Source: CAD feature listing. Evaluate the final solid. Frame: model axes, mm. A direction names the side the tool comes from. Coordinates: 2 decimals unless noted, no trailing zeros. Order: outer loops, then holes, each group sorted by start corner. A loop starts at its lowest first (then second) coordinate and runs counter-clockwise, first axis right, second up. Notation, with made-up numbers: (-27, 46) -> (7, 46) arc R13 cw to (7, 65) -> close; hole circle Ø11 at (-37.75, -30). An arc over 180 degrees is marked (long way). Write item = value, one per line. Start each with the question number.
Item 1: Contact query for flat-ended pins moving along their axis: pin 1 (6 mm diameter, centred on x = -4, z = -4, fed in from -Y); pin 2 (3 mm diameter, centred on x = 4, z = 4, fed in from -Y). Output: stop coordinate, or through.
Item 2: Section query C-C (x = -4). Output: boundary loops of the cut face in (y, z).
Item 3: Ray query, line 1 along X through (y, z) = (1.05, -4); line 2 along X through (y, z) = (1.05, 3.5); line 3 along Z through (x, y) = (-6, 1.4). Return the intervals inside material, ascending. Write a range as [from, to].
Item 4: Section query B-B (z = -4). Output: boundary loops of the cut face in (x, y).
Item 5: Set-up query: faces 4 (the cylindrical face through (-3.249, 0.887, 6.385)), 5 (the flat face through (0, 0, 0)). Return all of +Z, -Z, +X, -X, +Y, -Y with unobstructed straight access to the full face (end or side cutting, diameter ignored); none if empty.
Item 6: Section query A-A (y = 0.95). Output: boundary loops of the cut face in (x, z), then the cut area to 3 significant figures.
Item 7: Mould query, pull axis Z, two halves, no side actions, for faces 1 (the flat face through (0, 2, -7.9)), 2 (the flat face through (-7.9, 2, 0)), 3 (the cylindrical face through (-3.249, 0.887, -1.615)). Classes: released by +Z, released by -Z, zero draft, split by the parting line, or undercut.
```python
from build123d import *

# Parameters (mm, degrees)
SKETCH_1_W          = 15.8
SKETCH_1_H          = 15.8
SKETCH_1_R          = 2.5
EXTRUDE_1_DEPTH     = 3.2
SKETCH_1_5_R        = 2.5
CUT_EXTRUDE_1_DEPTH = 1.8


with BuildPart() as part:
    # Sketch 1 → Extrude 1 (new body)
    # profile 1 of 5: a face of its own
    with BuildSketch(Plane(origin=(0, 0, 0), x_dir=(1, 0, 0), z_dir=(0, 1, 0))):
        Rectangle(SKETCH_1_W, SKETCH_1_H)
        with Locations((4, -4)):
            Circle(SKETCH_1_R, mode=Mode.SUBTRACT)
        with Locations((-4, -4)):
            Circle(SKETCH_1_R, mode=Mode.SUBTRACT)
        with Locations((-4, 4)):
            Circle(SKETCH_1_R, mode=Mode.SUBTRACT)
        with Locations((4, 4)):
            Circle(SKETCH_1_R, mode=Mode.SUBTRACT)
    # profile 2 of 5: a face of its own
    with BuildSketch(Plane(origin=(0, 0, 0), x_dir=(1, 0, 0), z_dir=(0, 1, 0))):
        with Locations((4, -4)):
            Circle(SKETCH_1_R)
    # profile 3 of 5: a face of its own
    with BuildSketch(Plane(origin=(0, 0, 0), x_dir=(1, 0, 0), z_dir=(0, 1, 0))):
        with Locations((-4, -4)):
            Circle(SKETCH_1_R)
    # profile 4 of 5: a face of its own
    with BuildSketch(Plane(origin=(0, 0, 0), x_dir=(1, 0, 0), z_dir=(0, 1, 0))):
        with Locations((-4, 4)):
            Circle(SKETCH_1_R)
    # profile 5 of 5: a face of its own
    with BuildSketch(Plane(origin=(0, 0, 0), x_dir=(1, 0, 0), z_dir=(0, 1, 0))):
        with Locations((4, 4)):
            Circle(SKETCH_1_R)
    extrude(amount=EXTRUDE_1_DEPTH)

    # Sketch 1_5 → Cut-Extrude 1 (cut)
    with BuildSketch(Plane(origin=(0, 0, 0), x_dir=(1, 0, 0), z_dir=(0, 1, 0))):
        with Locations(Location((-4, -4, 0), (0, 0, 270))):
            Circle(SKETCH_1_5_R)
        with Locations(Location((4, -4, 0), (0, 0, 270))):
            Circle(SKETCH_1_5_R)
        with Locations(Location((4, 4, 0), (0, 0, 270))):
            Circle(SKETCH_1_5_R)
        with Locations(Location((-4, 4, 0), (0, 0, 270))):
            Circle(SKETCH_1_5_R)
    extrude(amount=CUT_EXTRUDE_1_DEPTH, mode=Mode.SUBTRACT)


solid = part.part
```
Computed:
q1.pin_1 = 0
q1.pin_2 = 1.8
q2.outline = (0, -7.9) -> (3.2, -7.9) -> (3.2, 7.9) -> (0, 7.9) -> (0, 6.5) -> (1.8, 6.5) -> (1.8, 1.5) -> (0, 1.5) -> (0, -1.5) -> (1.8, -1.5) -> (1.8, -6.5) -> (0, -6.5) -> close
q3.line_1 = [-7.9, -6.5], [-1.5, 1.5], [6.5, 7.9]
q3.line_2 = [-7.9, -6.45], [-1.55, 1.55], [6.45, 7.9]
q3.line_3 = [-7.9, -5.5], [-2.5, 2.5], [5.5, 7.9]
q4.outline = (-7.9, 0) -> (-6.5, 0) -> (-6.5, 1.8) -> (-1.5, 1.8) -> (-1.5, 0) -> (1.5, 0) -> (1.5, 1.8) -> (6.5, 1.8) -> (6.5, 0) -> (7.9, 0) -> (7.9, 3.2) -> (-7.9, 3.2) -> close
q5.face_4 = -Y
q5.face_5 = +Z, -Z, +X, -X, -Y
q6.outline = (-7.9, -7.9) -> (7.9, -7.9) -> (7.9, 7.9) -> (-7.9, 7.9) -> close; hole circle Ø5 at (-4, -4); hole circle Ø5 at (-4, 4); hole circle Ø5 at (4, -4); hole circle Ø5 at (4, 4)
q6.area = 171 mm^2
q7.face_1 = released by -Z
q7.face_2 = zero draft
q7.face_3 = undercut
